```python
from build123d import *
from build123d.topology import SkipClean

# Parameters (mm, degrees)
CORTE_R                 = 1.5
SALIENTE_EXTRUIR1_DEPTH = 3
SALIENTE_EXTRUIR2_START = -3
EXT1_R                  = 5.9
EXT1_R_2                = 2.75
SALIENTE_EXTRUIR2_DEPTH = 3
EXT2_R                  = 3
EXT2_R_2                = 1.5
SALIENTE_EXTRUIR3_DEPTH = 6


with BuildPart() as part:
    # Corte → Saliente-Extruir1 (new body)
    with BuildSketch(Plane.XY):
        with BuildLine():
            Line((35.929130783, 45.505192832), (60.592730783, 42.624770113))
            ThreePointArc((60.592730783, 42.624770113), (63.244730783, 39.645022473), (60.592730783, 36.665274833))
            Line((60.592730783, 36.665274833), (35.929130783, 33.784852114))
            ThreePointArc((35.929130783, 33.784852114), (29.344730783, 39.645022473), (35.929130783, 45.505192832))
        make_face()
        with Locations((35.244730783, 39.645022473)):
            Circle(CORTE_R, mode=Mode.SUBTRACT)
        with Locations((60.244730783, 39.645022473)):
            Circle(CORTE_R, mode=Mode.SUBTRACT)
    extrude(amount=SALIENTE_EXTRUIR1_DEPTH)

    # Ext1 → Saliente-Extruir2 (add)
    with SkipClean():  # the faces are left unmerged after this step: merging them gives an invalid solid
        with BuildSketch(Plane.XY.offset(SALIENTE_EXTRUIR2_START)):
            with Locations(Location((35.244730783, 39.645022473, 0), (0, 0, 83.338693133))):
                Circle(EXT1_R)
            with Locations((35.244730783, 39.645022473)):
                Circle(EXT1_R_2, mode=Mode.SUBTRACT)
        extrude(amount=SALIENTE_EXTRUIR2_DEPTH)

    # Ext2 → Saliente-Extruir3 (add)
    with SkipClean():  # the faces are left unmerged after this step: merging them gives an invalid solid
        with BuildSketch(Plane.XY):
            with Locations(Location((60.244730783, 39.645022473, 0), (0, 0, 83.338693133))):
                Circle(EXT2_R)
            with Locations((60.244730783, 39.645022473)):
                Circle(EXT2_R_2, mode=Mode.SUBTRACT)
        extrude(amount=SALIENTE_EXTRUIR3_DEPTH)


solid = part.part
```
Input: part model. Units: mm. Frame: model coordinates. A direction names the side the tool comes from. Coordinates: 2 decimals unless noted, no trailing zeros. Order: outer loops, then holes, each group sorted by start corner. A loop starts at its lowest first (then second) coordinate and runs counter-clockwise, first axis right, second up. Notation, with made-up numbers: (-8, 57.25) - (4, 57.25) arc R23 ccw to (4, 89.25) - close; hole circle Ø1 at (74, 83). An arc over 180 degrees is marked (long way). Put each result on its own line as item: value.
1. Draft query along Y for faces 1 (the face through (37.87, 40.47, -1.52)), 2 (the face through (48.088, 44.085, 1.479)), 3 (the face through (42, 40, 3)). Return one class per face: pulls with the +Y half, pulls with the -Y half, needs draft (parallel to the pull), parting line crosses it, or undercut.
Report:
face 1: undercut
face 2: pulls with the +Y half
face 3: needs draft
2. Cut plane C-C on y = 44.25. Return the cut outline in (x, z), then the cut area to 3 significant figures.
Report:
outline: (31.56, -3) - (38.93, -3) - (38.93, 0) - (46.68, 0) - (46.68, 3) - (31.56, 3) - close
area: 67.5 mm2
3. Reachability of faces 4 (the face through (61, 38, 6)), 5 (the face through (34, 38, 0)) from +Z, -Z, +X, -X, +Y, -Y: full face, straight path, thin tool, end or side. Return the list, or none.
Report:
face 4: +Z, +X, -X, +Y, -Y
face 5: -Z
4. Cut plane B-B on z = 5. Return the cut outline in (x, y), then the cut area to 3 significant figures.
Report:
outline: circle Ø6 at (60.24, 39.65); hole circle Ø3 at (60.24, 39.65)
area: 21.2 mm2
5. Cut plane D-D on x = 32. Return the cut outline in (y, z), then the cut area to 3 significant figures.
Report:
outline: (34.72, -3) - (44.57, -3) - (44.57, 3) - (34.72, 3) - close
area: 59.1 mm2
6. Contact query for flat-ended pins moving along their axis: pin 1 Ø3 at (x, y) = (35.5, 39.5) entering from -Z; pin 2 Ø4 at (x, y) = (50.5, 41) entering from +Z; pin 3 Ø3 at (y, z) = (42.5, 4) entering from +X. Output: stop coordinate, or through.
Report:
pin 1: stops at z = 0
pin 2: stops at z = 3
pin 3: stops at x = 62.92
7. Cut plane A-A on y = 38.5. Return the cut outline in (x, z), then the cut area to 3 significant figures.
Report:
outline: (29.46, -3) - (32.74, -3) - (32.74, 0) - (34.28, 0) - (34.28, 3) - (29.46, 3) - close; (36.21, 0) - (37.75, 0) - (37.75, -3) - (41.03, -3) - (41.03, 0) - (59.28, 0) - (59.28, 6) - (57.47, 6) - (57.47, 3) - (36.21, 3) - close; (61.21, 0) - (63.02, 0) - (63.02, 6) - (61.21, 6) - close
area: 120 mm2
8. Line query: line 1 along X through (y, z) = (39.5, 2.75); line 2 along X through (y, z) = (39.25, 2.5); line 3 along Z through (x, y) = (46, 40). Output: solid intervals per line, ascending.
Report:
line 1: x = 29.35 to 33.75, 36.74 to 58.75, 61.74 to 63.24
line 2: x = 29.36 to 33.8, 36.69 to 58.8, 61.69 to 63.22
line 3: z = 0 to 3
